from build123d import *

# Parameters (mm, degrees)
F0_R      = 14.75
F1_DEPTH  = 4.5
F2_R      = 2.8
F3_DEPTH  = 17
F4_R      = 2.3
F5_DEPTH  = 7
F3_FACE_R = 2.8
F6_DEPTH  = 5


with BuildPart() as f1:
    # F0 (on Right) → F1 (new body)
    with BuildSketch(Plane.YZ):
        Circle(F0_R)
    extrude(amount=F1_DEPTH)

    # F2 (on face) → F3 (join)
    with BuildSketch(Plane(origin=(0, 0, 0), x_dir=(0, -1, 0), z_dir=(-1, 0, 0))):
        Circle(F2_R)
    extrude(amount=F3_DEPTH)

    # F4 (on face) → F5 (join)
    with BuildSketch(Plane.YZ.offset(4.5)):
        with Locations((0, 10)):
            Circle(F4_R)
    extrude(amount=F5_DEPTH)

    # F3_face (on face) → F6 (join)
    with BuildSketch(Plane(origin=(-17, 0, 0), x_dir=(0, -1, 0), z_dir=(-1, 0, 0))):
        Circle(F3_FACE_R)
    extrude(amount=F6_DEPTH)


solid = f1.part
Verification items for the finished model (mm, model axes). A direction names the side the tool comes from. Round coordinates to 2 decimals unless told otherwise and drop trailing zeros. Loops run counter-clockwise (first coordinate to the right, second up) from the corner with the lowest first, then second, coordinate; pieces in that order, holes last. Notation, with made-up numbers: (-7, 32.25) - (27, 32.25) arc R25 ccw to (27, 66.25) - close; hole circle Ø1 at (13.5, 18.5). An arc over 180 degrees is marked (long way). Use a Markdown table: item, result. Add a question column.
1. Thickness scan on probe 1 along X at (y, z) = (-2.75, 5.5); probe 2 along X at (y, z) = (1, 9); probe 3 along Y at (x, z) = (1, 6). Record the ranges inside material, lowest first. Write a range as [from, to].
2. Section check D-D, the plane z = 11. Record the boundary of the cut face in (x, y).
3. Section check A-A, the plane z = 0. Record the boundary of the cut face in (x, y), plus the area to 3 significant figures.
4. Access from +Z, -Z, +X, -X, +Y, -Y to the whole of each face (thin tool, end or side, straight path). Record for faces 1 (the face through (7.95, -0.3, 12.28)), 2 (the face through (-10.8, 2.8, 0.1)), 3 (the face through (-22, 0, 0)).
5. Gauge pin test, flat ends, axial feed: pin 1 (1 mm diameter, centred on x = -15.5, z = -2, fed in from +Y); pin 2 (10 mm diameter, centred on y = -11, z = 1, fed in from +X); pin 3 (6 mm diameter, centred on y = 8, z = -7.5, fed in from -X). Record the tip position at first contact, or that the pin passes through.
6. Section check B-B, the plane y = 0. Record the boundary of the cut face in (x, z).
7. Section check C-C, the plane x = 9. Record the boundary of the cut face in (y, z), plus the area to 3 significant figures.
Checks:
| question | item | result |
|---|---|---|
| 1 | probe 1 | x = [0, 4.5] |
| 1 | probe 2 | x = [0, 11.5] |
| 1 | probe 3 | y = [-13.47, 13.47] |
| 2 | outline | (0, -9.83) - (4.5, -9.83) - (4.5, -2.07) - (11.5, -2.07) - (11.5, 2.07) - (4.5, 2.07) - (4.5, 9.83) - (0, 9.83) - close |
| 3 | outline | (-22, -2.8) - (0, -2.8) - (0, -14.75) - (4.5, -14.75) - (4.5, 14.75) - (0, 14.75) - (0, 2.8) - (-22, 2.8) - close |
| 3 | area | 256 mm^2 |
| 4 | face 1 | +X |
| 4 | face 2 | -X |
| 4 | face 3 | +Z, -Z, -X, +Y, -Y |
| 5 | pin 1 | stops at y = 2.36 |
| 5 | pin 2 | stops at x = 4.5 |
| 5 | pin 3 | stops at x = 0 |
| 6 | outline | (-22, -2.8) - (0, -2.8) - (0, -14.75) - (4.5, -14.75) - (4.5, 7.7) - (11.5, 7.7) - (11.5, 12.3) - (4.5, 12.3) - (4.5, 14.75) - (0, 14.75) - (0, 2.8) - (-22, 2.8) - close |
| 7 | outline | circle Ø4.6 at (0, 10) |
| 7 | area | 16.6 mm^2 |
